```python
from build123d import *

# Parameters (mm, degrees)
SKIZZE1_W                       = 61.8
SKIZZE1_H                       = 93.64
AUFSATZ_LINEAR_AUSTRAGEN1_DEPTH = 12
VERRUNDUNG1_R                   = 6
WANDUNG1_T                      = -1
SKIZZE2_W                       = 21.5
SKIZZE2_H                       = 17.5
SCHNITT_LINEAR_AUSTRAGEN1_DEPTH = 6
SKIZZE3_W                       = 22
SKIZZE3_H                       = 10
SCHNITT_LINEAR_AUSTRAGEN2_DEPTH = 6
SCHNITT_LINEAR_AUSTRAGEN4_DEPTH = 6
LINEARES_MUSTER1_COUNT          = 3
LINEARES_MUSTER1_PITCH          = 25
SKIZZE5_R                       = 2.5
AUFSATZ_LINEAR_AUSTRAGEN2_DEPTH = 3
SKIZZE6_R                       = 0.6
AUFSATZ_LINEAR_AUSTRAGEN3_DEPTH = 1


with BuildPart() as part:
    # Skizze1 → Aufsatz-Linear austragen1 (new body)
    with BuildSketch(Plane(origin=(0, 0, 0), x_dir=(0, 1, 0), z_dir=(0, 0, 1))):
        Rectangle(SKIZZE1_W, SKIZZE1_H)
    extrude(amount=AUFSATZ_LINEAR_AUSTRAGEN1_DEPTH)

    # Verrundung1
    verrundung1_edges = [part.edges().sort_by_distance(p)[0] for p in [
        (46.82, 30.9, 6),
        (46.82, -30.9, 6),
        (-46.82, -30.9, 6),
        (-46.82, 30.9, 6),
    ]]
    fillet(verrundung1_edges, radius=VERRUNDUNG1_R)

    # Wandung1
    wandung1_openings = [part.faces().sort_by_distance(p)[0] for p in [
        (0, 0, 12),
    ]]
    offset(amount=WANDUNG1_T, openings=wandung1_openings, kind=Kind.INTERSECTION)

    # Skizze2 → Schnitt-Linear austragen1 (cut)
    with BuildSketch(Plane.YZ.offset(46.82)):
        with Locations((0, 12)):
            Rectangle(SKIZZE2_W, SKIZZE2_H)
    extrude(amount=-SCHNITT_LINEAR_AUSTRAGEN1_DEPTH, mode=Mode.SUBTRACT)

    # Skizze3 → Schnitt-Linear austragen2 (cut)
    with BuildSketch(Plane.XZ.offset(30.9)):
        with Locations((-13.58, 7)):
            Rectangle(SKIZZE3_W, SKIZZE3_H)
    extrude(amount=-SCHNITT_LINEAR_AUSTRAGEN2_DEPTH, mode=Mode.SUBTRACT)

    # Skizze4 → Schnitt-Linear austragen4 (cut)
    with BuildSketch(Plane(origin=(0, 0, 0), x_dir=(1, 0, 0), z_dir=(0, 0, -1))):
        Polygon((-18.82, -2.339745962), (-28.82, -2.339745962), (-33.82, -11), (-28.82, -19.660254038), (-18.82, -19.660254038), (-13.82, -11), align=None)
    schnitt_linear_austragen4 = extrude(amount=-SCHNITT_LINEAR_AUSTRAGEN4_DEPTH, mode=Mode.SUBTRACT)

    # Lineares Muster1: Schnitt-Linear austragen4 ×3
    with Locations(*[(i * LINEARES_MUSTER1_PITCH, 0, 0) for i in range(1, LINEARES_MUSTER1_COUNT)]):
        add(schnitt_linear_austragen4, mode=Mode.SUBTRACT)

    # Skizze5 → Aufsatz-Linear austragen2 (add)
    with BuildSketch(Plane.XY.offset(1)):
        with Locations(Location((-34.19, 22.7, 0), (0, 0, 180))):
            Circle(SKIZZE5_R)
        with Locations(Location((39.65, 22.7, 0), (0, 0, 180))):
            Circle(SKIZZE5_R)
        with Locations(Location((39.65, -22.86, 0), (0, 0, 180))):
            Circle(SKIZZE5_R)
        with Locations(Location((-34.19, -22.86, 0), (0, 0, 180))):
            Circle(SKIZZE5_R)
    extrude(amount=AUFSATZ_LINEAR_AUSTRAGEN2_DEPTH)

    # Skizze6 → Aufsatz-Linear austragen3 (add)
    with BuildSketch(Plane.XY.offset(4)):
        with Locations((-34.19, 22.7)):
            Circle(SKIZZE6_R)
        with Locations((-34.19, -22.86)):
            Circle(SKIZZE6_R)
        with Locations((39.65, -22.86)):
            Circle(SKIZZE6_R)
        with Locations((39.65, 22.7)):
            Circle(SKIZZE6_R)
    extrude(amount=AUFSATZ_LINEAR_AUSTRAGEN3_DEPTH)


solid = part.part
```
Part model, mm, in its own coordinate system. A direction names the side the tool comes from. Give positions to 0.01 mm unless a question says otherwise; leave off trailing zeros. Loops run counter-clockwise (first coordinate to the right, second up) from the corner with the lowest first, then second, coordinate; pieces in that order, holes last. Notation, with made-up numbers: M 12,-27 L 62,-27 A20 cw 62,-17 Z; hole C 17.5,86 d9. An arc over 180 degrees is marked long. Return JSON: item names as keys, results as strings.
1) Saw through at D-D, the plane y = -3.5. List the corners of the cut face in (x, z).
Calculated:
{"outline": "M -46.82,0 L 46.82,0 L 46.82,3.25 L 45.82,3.25 L 45.82,1 L -45.82,1 L -45.82,12 L -46.82,12 Z"}
2) Saw through at C-C, the plane y = 4.5. List the corners of the cut face in (x, z), then the cut area to 3 significant figures.
Calculated:
{"outline": "M -46.82,0 L -30.07,0 L -30.07,1 L -45.82,1 L -45.82,12 L -46.82,12 Z; M -17.57,0 L -5.07,0 L -5.07,1 L -17.57,1 Z; M 7.43,0 L 19.93,0 L 19.93,1 L 7.43,1 Z; M 32.43,0 L 46.82,0 L 46.82,3.25 L 45.82,3.25 L 45.82,1 L 32.43,1 Z", "area": "69.4 mm2"}
3) Saw through at B-B, the plane z = 7.25. List the corners of the cut face in (x, y), then the cut area to 3 significant figures.
Calculated:
{"outline": "M -46.82,-24.9 A6 ccw -40.82,-30.9 L -24.58,-30.9 L -24.58,-29.9 L -40.82,-29.9 A5 cw -45.82,-24.9 L -45.82,24.9 A5 cw -40.82,29.9 L 40.82,29.9 A5 cw 45.82,24.9 L 45.82,10.75 L 46.82,10.75 L 46.82,24.9 A6 ccw 40.82,30.9 L -40.82,30.9 A6 ccw -46.82,24.9 Z; M -2.58,-30.9 L 40.82,-30.9 A6 ccw 46.82,-24.9 L 46.82,-10.75 L 45.82,-10.75 L 45.82,-24.9 A5 cw 40.82,-29.9 L -2.58,-29.9 Z", "area": "254 mm2"}
4) Pull direction Y, two halves, no side cores. Call faces 4 (the face through (-44.32, -28.47, 6.58)), 5 (the face through (-45.016, -29.189, 6.084)), 6 (the face through (1, 30.9, 6)): released by +Y, released by -Y, zero draft, split by the parting line, or undercut.
Calculated:
{"face 4": "undercut", "face 5": "released by -Y", "face 6": "released by +Y"}
5) Flat gauge pins, fed straight in: pin 1 Ø1.5 at (x, y) = (-33.5, 23) entering from +Z; pin 2 Ø1.1 at (y, z) = (-30.5, 5.5) entering from +X; pin 3 Ø0.8 at (x, y) = (-15.5, -30.5) entering from +Z; pin 4 Ø12 at (x, y) = (24, 11) entering from -Z. Where does each tip first touch, or does it go through?
Calculated:
{"pin 1": "stops at z = 5", "pin 2": "stops at x = 44.06", "pin 3": "stops at z = 2", "pin 4": "passes through"}
6) 3-axis set-ups, long thin cutter, end or side, ignore diameter. For faces 1 (the face through (33.645, 15.391, 0.493)), 2 (the face through (-35, 23, 4)), 3 (the face through (45.109, 29.096, 6.084)): which of +Z, -Z, +X, -X, +Y, -Y reach the whole face in a straight line?
Calculated:
{"face 1": "+Z, -Z", "face 2": "+Z", "face 3": "+Z, -Z, +X, +Y"}
7) Saw through at A-A, the plane x = 3.5. List the corners of the cut face in (y, z), then the cut area to 3 significant figures.
Calculated:
{"outline": "M -30.9,0 L 2.34,0 L 2.34,1 L -29.9,1 L -29.9,12 L -30.9,12 Z; M 19.66,0 L 30.9,0 L 30.9,12 L 29.9,12 L 29.9,1 L 19.66,1 Z", "area": "66.5 mm2"}
8) Drill centre lines: line 1 (Y direction, x = -41, z = 7.75); line 2 (Y direction, x = 1, z = 0.75); line 3 (X direction, y = 25, z = 1.25). Where is each one in solid material? Low to high.
Calculated:
{"line 1": "y = -30.9 to -29.9, 29.9 to 30.9", "line 2": "y = -30.9 to 2.34, 19.66 to 30.9", "line 3": "x = -46.82 to -45.82, -35.17 to -33.21, 38.67 to 40.63, 45.82 to 46.82"}
